The listing builds one solid part. Answer for the finished solid, in the listing's coordinates (mm). Face numbers are marked on the shaded views. A direction names the side the tool comes from. Give positions to 0.01 mm unless a question says otherwise; leave off trailing zeros. Order: outer loops, then holes, each group sorted by start corner. A loop starts at its lowest first (then second) coordinate and runs counter-clockwise, first axis right, second up. Notation, with made-up numbers: (61.25, 25.25) -> (111.25, 25.25) arc R32 cw to (111.25, 62.25) -> close; hole circle Ø10 at (80, 54.25). An arc over 180 degrees is marked (long way). One line per question, with ' | ' between items. Start each with the question number.
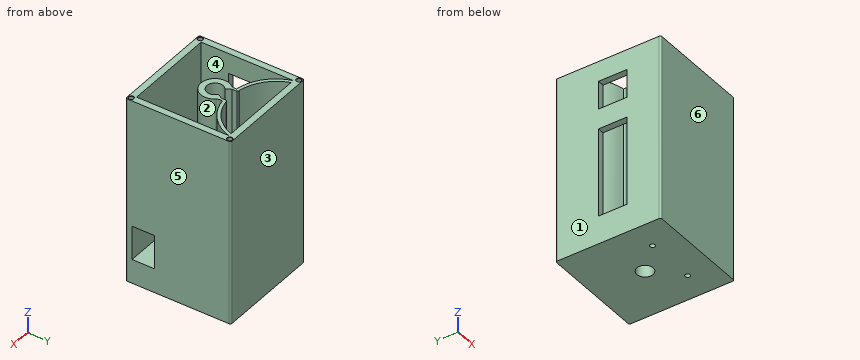
Autodesk Inventor part; units mm, degrees
ref_plane "YZ Plane" through (0, 0, 0) normal (1, 0, 0) x (0, 1, 0)
ref_plane "XZ Plane" through (0, 0, 0) normal (0, 1, 0) x (-1, 0, 0)
ref_plane "XY Plane" through (0, 0, 0) normal (0, 0, 1) x (1, 0, 0)
sketch "Sketch1" plane through (0, 0, 0) normal (0, 0, 1) x (1, 0, 0)
  circle A0 centre (0, 0) radius 5
  line L0 (15.5, -15.5) -> (-15.5, -15.5) construction
  line L1 (-15.5, -15.5) -> (-15.5, 15.5) construction
  line L2 (-15.5, 15.5) -> (15.5, 15.5) construction
  line L3 (15.5, 15.5) -> (15.5, -15.5) construction
  line L4 (15.5, -15.5) -> (-15.5, 15.5) construction
  line L5 (-15.5, -15.5) -> (15.5, 15.5) construction
  circle A1 centre (-15.5, 15.5) radius 1.5
  circle A2 centre (15.5, 15.5) radius 1.5
  circle A3 centre (15.5, -15.5) radius 1.5
  circle A4 centre (-15.5, -15.5) radius 1.5
  line L6 (31.5, -32.5) -> (-31.5, -32.5)
  line L7 (-32.5, -31.5) -> (-32.5, 31.5)
  line L8 (-31.5, 32.5) -> (31.5, 32.5)
  line L9 (32.5, 31.5) -> (32.5, -31.5)
  line L10 (32.5, -32.5) -> (-32.5, 32.5) construction
  line L11 (-32.5, -32.5) -> (32.5, 32.5) construction
  arc A5 (-31.5, 32.5) -> (-32.5, 31.5) centre (-31.5, 31.5) ccw
  arc A6 (-32.5, -31.5) -> (-31.5, -32.5) centre (-31.5, -31.5) ccw
  arc A7 (31.5, -32.5) -> (32.5, -31.5) centre (31.5, -31.5) ccw
  arc A8 (32.5, 31.5) -> (31.5, 32.5) centre (31.5, 31.5) ccw
  arc A9 (-6.8415, 5.4549) -> (6.8415, 5.4549) centre (0, 0) ccw
  line L12 (-6.1872, 7.3252) -> (-6.1872, 8.9372)
  line L13 (-6.1872, 8.9372) -> (6.1872, 8.9372)
  line L14 (6.1872, 8.9372) -> (6.1872, 7.3252)
  arc A10 (-6.8415, 5.4549) -> (-6.1872, 7.3252) centre (-9.1872, 7.3252) ccw
  arc A11 (6.1872, 7.3252) -> (6.8415, 5.4549) centre (9.1872, 7.3252) ccw
  line L15 (28.5, 28.5) -> (-28.5, 28.5)
  line L16 (-28.5, 28.5) -> (-28.5, -28.5)
  line L17 (-28.5, -28.5) -> (28.5, -28.5)
  line L18 (28.5, -28.5) -> (28.5, 28.5)
  point P0 (-6.1872, 6.1872)
  point P1 (6.1872, 6.1872)
  dimension "d0" = 10
  dimension "d1" = 31
  dimension "d2" = 31
  dimension "d3" = 3
  dimension "d4" = 3
  dimension "d5" = 3
  dimension "d6" = 3
  dimension "d7" = 65
  dimension "d8" = 65
  dimension "d9" = 1
  dimension "d10" = 17.5
  dimension "d11" = 2.75
  dimension "d12" = 3
  dimension "d13" = 4
extrude "Extrusion1" add sketch "Sketch1" along normal blind 115 contours L6 A6 L7 A5 L8 A8 L9 A7 | A10 L12 L13 L14 A11 A9
extrude "Extrusion2" add sketch "Sketch1" along normal blind 15 contours L18 L17 L16 L15
sketch "Sketch2" plane through (-31.5, 32.5, 0) normal (0, 1, 0) x (1, 0, 0)
  point P0 (31.5, 0)
sketch "Sketch3" plane through (0, 0, 115) normal (0, 0, 1) x (1, 0, 0)
  arc A0 (-28.5, 28.5) -> (-6.1872, 8.9372) centre (-2.0793, 36.1286) ccw
  line L0 (6.1872, 7.3252) -> (6.1872, 8.9372)
  line L1 (28.5, 28.5) -> (28.5, -28.5)
  arc A1 (6.1872, 8.9372) -> (28.5, 28.5) centre (2.0793, 36.1286) ccw
  line L2 (6.1872, 8.9372) -> (-6.1872, 8.9372)
  line L3 (-28.5, 28.5) -> (28.5, 28.5)
  line L4 (-28.5, 28.5) -> (-26.5, 28.5)
  line L5 (28.5, 28.5) -> (26.5, 28.5)
  arc A2 (-26.5, 28.5) -> (-6.1872, 10.9372) centre (-1.4006, 37.0013) ccw
  arc A3 (6.1872, 10.9372) -> (26.5, 28.5) centre (1.4006, 37.0013) ccw
  line L6 (-6.1872, 8.9372) -> (-6.1872, 7.3252)
  line L7 (-6.1872, 8.9372) -> (-6.1872, 7.3252)
  line L8 (-6.1872, 7.3252) -> (-4.6872, 7.3252)
  line L9 (-4.6872, 7.3252) -> (-4.6872, 10.1872)
  line L10 (6.1872, 8.9372) -> (6.1872, 7.3252)
  line L11 (6.1872, 7.3252) -> (4.6872, 7.3252)
  line L12 (4.6872, 7.3252) -> (4.6872, 10.1872)
  line L13 (-6.1872, 10.9372) -> (-5.4372, 10.9372)
  line L14 (5.4372, 10.9372) -> (6.1872, 10.9372)
  line L15 (-4.6872, 10.1872) -> (-5.4372, 10.9372)
  line L16 (4.6872, 10.1872) -> (5.4372, 10.9372)
  line L17 (-5.4372, 10.9372) -> (5.4372, 10.9372)
  line L18 (4.6872, 7.3252) -> (-4.6872, 7.3252)
  line L19 (-4.6872, 7.3252) -> (-2.8356, 4.1182)
  line L20 (-4.6872, 7.3252) -> (-0.7761, 7.3252) construction
  line L21 (4.6872, 7.1776) -> (8.8154, 7.1776) construction
  circle A4 centre (0, 0) radius 5
  line L22 (4.6872, 7.3252) -> (2.8356, 4.1182)
  line L23 (4.6872, 7.3252) -> (9.2305, 7.3252) construction
  circle A5 centre (0, 0) radius 8.75
  point P0 (-4.6872, 10.9372)
  point P1 (4.6872, 10.9372)
  point P2 (-4.7858, 7.3252)
  point P3 (-4.6872, 7.3887)
  point P4 (4.6872, 7.3887)
  point P5 (4.7858, 7.3252)
  dimension "d18" = 27.5
  dimension "d19" = 27.5
  dimension "d20" = 2
  dimension "d21" = 2
  dimension "d23" = 26.5
  dimension "d24" = 26.5
  dimension "d25" = 22.3128
  dimension "d26" = 29.9006
  dimension "d27" = 1.5
  dimension "d28" = 1.5
  dimension "d29" = 2
  dimension "d30" = 2
  dimension "d31" = 0.75
  dimension "d32" = 0.75
  dimension "d33" = 0.75
  dimension "d34" = 0.75
  dimension "d35" = 60
  dimension "d37" = 120
  dimension "d38" = 10
  dimension "d39" = 17.5
extrude "Extrusion3" add sketch "Sketch3" against normal blind 105 contours L3 A2 L13 L15 L9 L2 A0 | L2 L9 A5 L8 L6 | L3 A1 L2 L12 L16 L14 A3 | L2 L0 L11 A5 L12
extrude "Extrusion4" cut sketch "Sketch3" against normal blind 80 contours L9 L15 L17 L16 L12 L2 | L2 L12 A5 L9 | A5 L12 L18 L9 | L18 L22 A4 L19
extrude "Extrusion5" add sketch "Sketch1" along normal blind 15 contours A1 | A2
chamfer "Chamfer1" distance 2 angle 45 1 edges at (0, 8.9372, 35)
sketch "Sketch4" plane through (0, 0, 115) normal (0, 0, 1) x (1, 0, 0)
  line L0 (30.5, -30.5) -> (-30.5, -30.5) construction
  line L1 (-30.5, -30.5) -> (-30.5, 30.5) construction
  line L2 (-30.5, 30.5) -> (30.5, 30.5) construction
  line L3 (30.5, 30.5) -> (30.5, -30.5) construction
  line L4 (30.5, -30.5) -> (-30.5, 30.5) construction
  line L5 (-30.5, -30.5) -> (30.5, 30.5) construction
  circle A0 centre (-30.5, 30.5) radius 1.45
  circle A1 centre (30.5, 30.5) radius 1.45
  circle A2 centre (30.5, -30.5) radius 1.45
  circle A3 centre (-30.5, -30.5) radius 1.45
  point P0 (0, 0)
  dimension "d52" = 61
  dimension "d53" = 61
  dimension "d54" = 2.9
  dimension "d55" = 2.9
  dimension "d56" = 2.9
  dimension "d57" = 2.9
extrude "Extrusion6" cut sketch "Sketch4" against normal blind 60
chamfer "Chamfer2" distance 0.2 angle 45 6 edges at (-31.95, 30.5, 115) (29.05, 30.5, 115) (-31.95, -30.5, 115) (-17, -15.5, 15) (14, -15.5, 15) (29.05, -30.5, 115)
sketch "Sketch5" plane through (-32.5, -31.5, 0) normal (-1, 0, 0) x (0, 0, 1)
  line L0 (17.5, 37.5) -> (72.5, 37.5)
  line L1 (72.5, 37.5) -> (72.5, 20)
  line L2 (72.5, 20) -> (17.5, 20)
  line L3 (17.5, 20) -> (17.5, 37.5)
  line L4 (85, 37.5) -> (102.5, 37.5)
  line L5 (102.5, 37.5) -> (102.5, 20)
  line L6 (102.5, 20) -> (85, 20)
  line L7 (85, 20) -> (85, 37.5)
  line L8 (0, 63) -> (0, 0)
  line L9 (115, 63) -> (115, 0)
  point P0 (0, 31.5)
  dimension "d63" = 12.5
  dimension "d64" = 17.5
  dimension "d65" = 17.5
  dimension "d66" = 55
  dimension "d67" = 12.5
  dimension "d68" = 20
extrude "Extrusion7" cut sketch "Sketch5" against normal up to surface (4 mm away)
sketch "Sketch6" plane through (32.5, -31.5, 0) normal (1, 0, 0) x (0, 0, -1)
  line L0 (-15, 60) -> (-15, 3)
  line L1 (-15, 3) -> (-36, 3)
  line L2 (-36, 3) -> (-36, 17)
  line L3 (-36, 17) -> (-15, 17)
  line L4 (-15, 17) -> (-15, 3)
  point P0 (0, 31.5)
  dimension "d71" = 21
  dimension "d72" = 14
extrude "Extrusion8" cut sketch "Sketch6" against normal up to surface (4 mm away)
equation "\"d5\" = d4"
equation "\"d6\" = d5"
properties part number "doser-housing"
(1) For the marked faces 1 and 2, determine the directions among +Z, -Z, +X, -X, +Y, -Y from which every point of the face is accessible in a straight line to the end or side of a thin tool.
(2) Consider line 1 (X direction, y = 0, z = 26); line 2 (Y direction, x = -30.5, z = 82.5); line 3 (X direction, y = -30, z = 96). Determine where each line is inside the solid, lowest interval first.
(3) The part is cut by section C-C on y = -3.5. Determine the outline of the cut face in (x, z), plus the area to 3 significant figures.
(4) The part is cut by section D-D on x = -12. Determine the outline of the cut face in (y, z), plus the area to 3 significant figures.
(5) Determine the mould class of the marked faces 3, 4, 5 and 6 for opening direction Y: pulls with the +Y half, pulls with the -Y half, needs draft (parallel to the pull), parting line crosses it, or undercut.
(6) The part is cut by section B-B on z = 19.5. State how many separate pieces and enclosed holes the cut face has, plus the area to 3 significant figures.
(7) The part is cut by section A-A on x = 0. Determine the outline of the cut face in (y, z), plus the area to 3 significant figures.
(8) Given P1, Ø1.4, axis at x = 30.5, y = 30.5, coming from the +Z side; P2, Ø2, axis at x = 24.5, y = -15, coming from the +Z side; P3, Ø3, axis at x = -1.5, y = 5, coming from the +Z side; P4, Ø10, axis at x = -25, y = -17, coming from the -Z side, each flat-ended and moving along its own axis, determine where each tip first touches the part or whether it passes through.
Result sheet:
1) face 1: +Z, -Z, -X, +Y, -Y | face 2: +Z
2) line 1: x = -8.75 to -5, 5 to 8.75, 28.5 to 32.5 | line 2: y = -32.5 to -31.95, -29.05 to 29.05, 31.95 to 32.5 | line 3: x = -32.5 to -31.86, -29.14 to 29.14, 31.86 to 32.5
3) outline: (-32.5, 0) -> (-3.57, 0) -> (-3.57, 115) -> (-8.02, 115) -> (-8.02, 15) -> (-28.5, 15) -> (-28.5, 17.5) -> (-32.5, 17.5) -> close; (-32.5, 72.5) -> (-28.5, 72.5) -> (-28.5, 85) -> (-32.5, 85) -> close; (-32.5, 102.5) -> (-28.5, 102.5) -> (-28.5, 115) -> (-32.5, 115) -> close; (3.57, 0) -> (32.5, 0) -> (32.5, 115) -> (28.5, 115) -> (28.5, 15) -> (8.02, 15) -> (8.02, 115) -> (3.57, 115) -> close | area: 2,270 mm^2
4) outline: (-32.5, 0) -> (32.5, 0) -> (32.5, 115) -> (28.5, 115) -> (28.5, 15) -> (12.71, 15) -> (12.71, 115) -> (10.48, 115) -> (10.48, 15) -> (-28.5, 15) -> (-28.5, 115) -> (-32.5, 115) -> close | area: 2,000 mm^2
5) face 3: pulls with the +Y half | face 4: undercut | face 5: needs draft | face 6: pulls with the -Y half
6) separate pieces: 2 | enclosed holes: 2 | area: 1,150 mm^2
7) outline: (-32.5, 0) -> (-5, 0) -> (-5, 115) -> (-8.75, 115) -> (-8.75, 15) -> (-28.5, 15) -> (-28.5, 115) -> (-32.5, 115) -> close; (5, 0) -> (32.5, 0) -> (32.5, 115) -> (28.5, 115) -> (28.5, 15) -> (8.94, 15) -> (8.94, 33) -> (6.94, 35) -> (5, 35) -> close | area: 2,080 mm^2
8) P1: stops at z = 55 | P2: stops at z = 15 | P3: stops at z = 35 | P4: stops at z = 0
